For this review, use the dimensioned drawing (mm, ordinates from the lowest corner) and the shaded views. Coordinates: 2 decimals unless noted, no trailing zeros. Loops run counter-clockwise (first coordinate to the right, second up) from the corner with the lowest first, then second, coordinate; pieces in that order, holes last. Notation, with made-up numbers: (2, 56) - (31, 56) arc R35 cw to (31, 92) - close; hole circle Ø4 at (-36, 18.25). An arc over 180 degrees is marked (long way). Answer in a Markdown table with one row per item. Add a question column.
(1) Clearance check with flat-ended pins moving along their axes: pin 1 (5 mm diameter, centred on x = 12.5, y = 147.5, fed in from +Z); pin 2 (11.5 mm diameter, centred on y = 665, z = 125, fed in from -X). State where each tip first meets the part, or that it passes through.
(2) We need section A-A, the plane y = 485. Write out the cut boundary in (x, z).
(3) We need section B-B, the plane z = 75. Write out the cut boundary in (x, y), plus the area to 3 significant figures.
(4) We need section C-C, the plane x = 13. Give the number of separate pieces and of enclosed holes in the cut face, plus the area to 3 significant figures.
(5) To check wall thickness, follow L1, parallel to Y at x = 8.75, z = 76; L2, parallel to Z at x = 8.5, y = 505; L3, parallel to Y at x = 6, z = 75. State the ranges of each line that lie inside material, in increasing order. Write a range as [from, to].
(6) We need section D-D, the plane z = 125. Write out the cut boundary in (x, y).
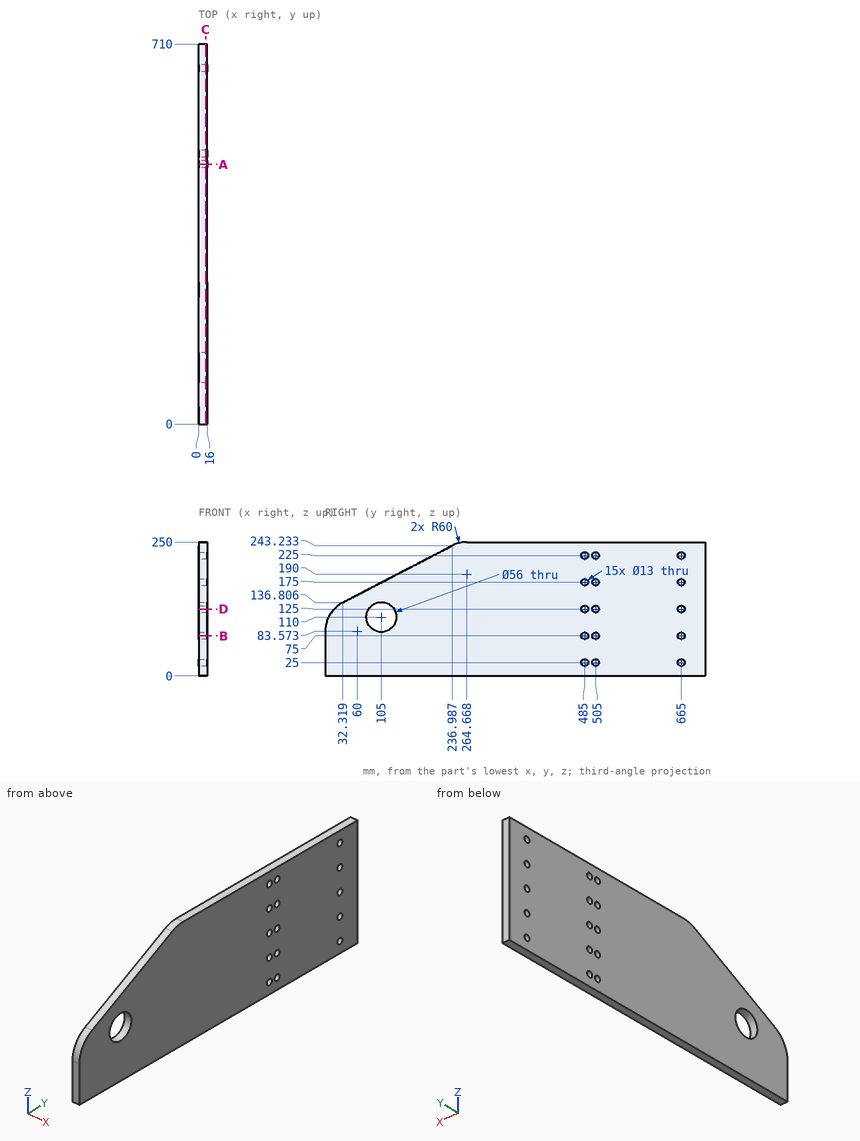
Responses:
| question | item | result |
|---|---|---|
| 1 | pin 1 | stops at z = 198 |
| 1 | pin 2 | passes through |
| 2 | outline | (0, 0) - (16, 0) - (16, 18.5) - (0, 18.5) - close; (0, 31.5) - (16, 31.5) - (16, 68.5) - (0, 68.5) - close; (0, 81.5) - (16, 81.5) - (16, 118.5) - (0, 118.5) - close; (0, 131.5) - (16, 131.5) - (16, 168.5) - (0, 168.5) - close; (0, 181.5) - (16, 181.5) - (16, 218.5) - (0, 218.5) - close; (0, 231.5) - (16, 231.5) - (16, 250) - (0, 250) - close |
| 3 | outline | (0, 0) - (16, 0) - (16, 478.5) - (0, 478.5) - close; (0, 491.5) - (16, 491.5) - (16, 498.5) - (0, 498.5) - close; (0, 511.5) - (16, 511.5) - (16, 658.5) - (0, 658.5) - close; (0, 671.5) - (16, 671.5) - (16, 710) - (0, 710) - close |
| 3 | area | 10,700 mm2 |
| 4 | separate pieces | 1 |
| 4 | enclosed holes | 16 |
| 4 | area | 157,000 mm2 |
| 5 | L1 | y = [0, 478.58], [491.42, 498.58], [511.42, 658.58], [671.42, 710] |
| 5 | L2 | z = [0, 18.5], [31.5, 68.5], [81.5, 118.5], [131.5, 168.5], [181.5, 218.5], [231.5, 250] |
| 5 | L3 | y = [0, 478.5], [491.5, 498.5], [511.5, 658.5], [671.5, 710] |
| 6 | outline | (0, 16.6) - (16, 16.6) - (16, 81.36) - (0, 81.36) - close; (0, 128.64) - (16, 128.64) - (16, 478.5) - (0, 478.5) - close; (0, 491.5) - (16, 491.5) - (16, 498.5) - (0, 498.5) - close; (0, 511.5) - (16, 511.5) - (16, 658.5) - (0, 658.5) - close; (0, 671.5) - (16, 671.5) - (16, 710) - (0, 710) - close |
